```python
from build123d import *

# Parameters (mm, degrees)
F1_DEPTH = 4
F3_DEPTH = 2.5
F4_R     = 4
F5_DEPTH = 1
F6_R     = 1.75
F7_DEPTH = 5.001
F8_SIZE  = 0.99999


# Not quite as in the source:
# - a fillet or chamfer is up to 0.001 mm smaller than in the source, because OpenCascade refuses the exact size


with BuildPart() as f1:
    # F0 (on Top) → F1 (new body)
    with BuildSketch(Plane.XY):
        with BuildLine():
            ThreePointArc((-1.75, 7.5042031676), (-1.8060506469, 7.3388969595), (-1.9510840407, 7.2417726467))
            ThreePointArc((-1.9510840407, 7.2417726467), (-3.75, 6.4951905284), (-5.2960170601, 5.3105746675))
            ThreePointArc((-5.2960170601, 5.3105746675), (-5.4526458792, 5.2335342205), (-5.6238305783, 5.2676460404))
            Line((-5.6238305783, 5.2676460404), (-5.7871696323, 5.3619498872))
            ThreePointArc((-5.7871696323, 5.3619498872), (-6.3349564147, 5.8273689108), (-6.682813556, 6.4564004169))
            ThreePointArc((-6.682813556, 6.4564004169), (-12.124355653, 7), (-8.932813556, 2.5592860998))
            ThreePointArc((-8.932813556, 2.5592860998), (-8.2141277213, 2.5725487316), (-7.5371696323, 2.330860974))
            Line((-7.5371696323, 2.330860974), (-7.3738305783, 2.2365571272))
            ThreePointArc((-7.3738305783, 2.2365571272), (-7.2586965261, 2.105362739), (-7.2471011008, 1.9311979792))
            ThreePointArc((-7.2471011008, 1.9311979792), (-7.5, 0), (-7.2471011008, -1.9311979792))
            ThreePointArc((-7.2471011008, -1.9311979792), (-7.2586965261, -2.105362739), (-7.3738305783, -2.2365571272))
            Line((-7.3738305783, -2.2365571272), (-7.5371696323, -2.330860974))
            ThreePointArc((-7.5371696323, -2.330860974), (-8.2141277213, -2.5725487316), (-8.932813556, -2.5592860998))
            ThreePointArc((-8.932813556, -2.5592860998), (-12.124355653, -7), (-6.682813556, -6.4564004169))
            ThreePointArc((-6.682813556, -6.4564004169), (-6.3349564147, -5.8273689108), (-5.7871696323, -5.3619498872))
            Line((-5.7871696323, -5.3619498872), (-5.6238305783, -5.2676460404))
            ThreePointArc((-5.6238305783, -5.2676460404), (-5.4526458792, -5.2335342205), (-5.2960170601, -5.3105746675))
            ThreePointArc((-5.2960170601, -5.3105746675), (-3.75, -6.4951905284), (-1.9510840407, -7.2417726467))
            ThreePointArc((-1.9510840407, -7.2417726467), (-1.8060506469, -7.3388969595), (-1.75, -7.5042031676))
            Line((-1.75, -7.5042031676), (-1.75, -7.6928108612))
            ThreePointArc((-1.75, -7.6928108612), (-1.8791713066, -8.3999176424), (-2.25, -9.0156865167))
            ThreePointArc((-2.25, -9.0156865167), (0, -14), (2.25, -9.0156865167))
            ThreePointArc((2.25, -9.0156865167), (1.8791713066, -8.3999176424), (1.75, -7.6928108612))
            Line((1.75, -7.6928108612), (1.75, -7.5042031676))
            ThreePointArc((1.75, -7.5042031676), (1.8060506469, -7.3388969595), (1.9510840407, -7.2417726467))
            ThreePointArc((1.9510840407, -7.2417726467), (3.75, -6.4951905284), (5.2960170601, -5.3105746675))
            ThreePointArc((5.2960170601, -5.3105746675), (5.4526458792, -5.2335342205), (5.6238305783, -5.2676460404))
            Line((5.6238305783, -5.2676460404), (5.7871696323, -5.3619498872))
            ThreePointArc((5.7871696323, -5.3619498872), (6.3349564147, -5.8273689108), (6.682813556, -6.4564004169))
            ThreePointArc((6.682813556, -6.4564004169), (12.124355653, -7), (8.932813556, -2.5592860998))
            ThreePointArc((8.932813556, -2.5592860998), (8.2141277213, -2.5725487316), (7.5371696323, -2.330860974))
            Line((7.5371696323, -2.330860974), (7.3738305783, -2.2365571272))
            ThreePointArc((7.3738305783, -2.2365571272), (7.2586965261, -2.105362739), (7.2471011008, -1.9311979792))
            ThreePointArc((7.2471011008, -1.9311979792), (7.5, 0), (7.2471011008, 1.9311979792))
            ThreePointArc((7.2471011008, 1.9311979792), (7.2586965261, 2.105362739), (7.3738305783, 2.2365571272))
            Line((7.3738305783, 2.2365571272), (7.5371696323, 2.330860974))
            ThreePointArc((7.5371696323, 2.330860974), (8.2141277213, 2.5725487316), (8.932813556, 2.5592860998))
            ThreePointArc((8.932813556, 2.5592860998), (12.124355653, 7), (6.682813556, 6.4564004169))
            ThreePointArc((6.682813556, 6.4564004169), (6.3349564147, 5.8273689108), (5.7871696323, 5.3619498872))
            Line((5.7871696323, 5.3619498872), (5.6238305783, 5.2676460404))
            ThreePointArc((5.6238305783, 5.2676460404), (5.4526458792, 5.2335342205), (5.2960170601, 5.3105746675))
            ThreePointArc((5.2960170601, 5.3105746675), (3.75, 6.4951905284), (1.9510840407, 7.2417726467))
            ThreePointArc((1.9510840407, 7.2417726467), (1.8060506469, 7.3388969595), (1.75, 7.5042031676))
            Line((1.75, 7.5042031676), (1.75, 7.6928108612))
            ThreePointArc((1.75, 7.6928108612), (1.8791713066, 8.3999176424), (2.25, 9.0156865167))
            ThreePointArc((2.25, 9.0156865167), (0, 14), (-2.25, 9.0156865167))
            ThreePointArc((-2.25, 9.0156865167), (-1.8791713066, 8.3999176424), (-1.75, 7.6928108612))
            Line((-1.75, 7.6928108612), (-1.75, 7.5042031676))
        make_face()
    extrude(amount=F1_DEPTH)

    # F2 (on Top) → F3 (cut)
    with BuildSketch(Plane.XY):
        Polygon((2.875, -1.6598820239), (2.875, 1.6598820239), (0, 3.3197640478), (-2.875, 1.6598820239), (-2.875, -1.6598820239), (0, -3.3197640478), align=None)
    extrude(amount=F3_DEPTH, mode=Mode.SUBTRACT)

    # F4 (on face) → F5 (join)
    with BuildSketch(Plane.XY.offset(4)):
        Circle(F4_R)
    extrude(amount=F5_DEPTH)

    # F6 (on face) → F7 (cut, through all)
    with BuildSketch(Plane.XY.offset(5)):
        Circle(F6_R)
    extrude(amount=-F7_DEPTH, mode=Mode.SUBTRACT)

    # F8 (size 1 in the source; OpenCascade refuses exactly that, so slightly less here)
    f8_edges = [f1.edges().sort_by_distance(p)[0] for p in [
        (1.75, -7.598507, 4),
        (1.879171, -8.399918, 4),
        (1.806051, -7.338897, 4),
        (0, -14, 4),
        (3.75, -6.495191, 4),
        (-1.879171, -8.399918, 4),
        (5.452646, -5.233534, 4),
        (-1.75, -7.598507, 4),
        (5.7055, -5.314798, 4),
        (-1.806051, -7.338897, 4),
        (6.334956, -5.827369, 4),
        (-3.75, -6.495191, 4),
        (12.124356, -7, 4),
        (-5.452646, -5.233534, 4),
        (8.214128, -2.572549, 4),
        (-5.7055, -5.314798, 4),
        (7.4555, -2.283709, 4),
        (-6.334956, -5.827369, 4),
        (7.258697, -2.105363, 4),
        (-12.124356, -7, 4),
        (7.5, 0, 4),
        (-8.214128, -2.572549, 4),
        (7.258697, 2.105363, 4),
        (-7.4555, -2.283709, 4),
        (7.4555, 2.283709, 4),
        (-7.258697, -2.105363, 4),
        (8.214128, 2.572549, 4),
        (-7.5, 0, 4),
        (12.124356, 7, 4),
        (-7.258697, 2.105363, 4),
        (6.334956, 5.827369, 4),
        (-7.4555, 2.283709, 4),
        (5.7055, 5.314798, 4),
        (-8.214128, 2.572549, 4),
        (5.452646, 5.233534, 4),
        (-12.124356, 7, 4),
        (3.75, 6.495191, 4),
        (-6.334956, 5.827369, 4),
        (1.806051, 7.338897, 4),
        (-5.7055, 5.314798, 4),
        (1.75, 7.598507, 4),
        (-5.452646, 5.233534, 4),
        (1.879171, 8.399918, 4),
        (-3.75, 6.495191, 4),
        (0, 14, 4),
        (-1.806051, 7.338897, 4),
        (-1.879171, 8.399918, 4),
        (-1.75, 7.598507, 4),
        (-4, 0, 4),
        (-12.124356, -7, 0),
    ]]
    chamfer(f8_edges, length=F8_SIZE)


solid = f1.part
```
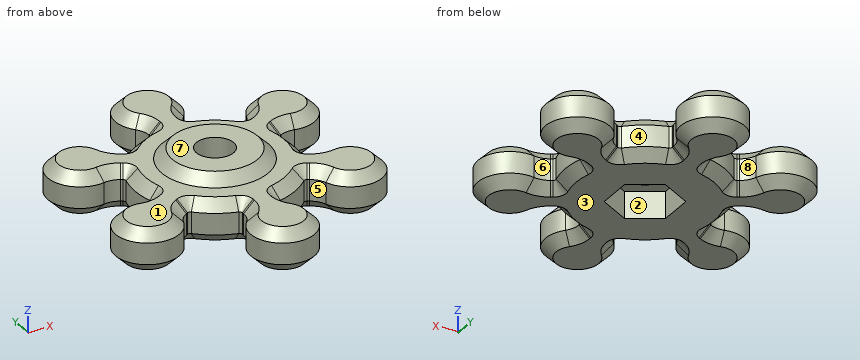
The model under review builds one solid part; all positions refer to its coordinate system, in mm. Face numbers are marked on the shaded views. A direction names the side the tool comes from. Coordinates: 2 decimals unless noted, no trailing zeros. Write each loop counter-clockwise with the first axis right and the second up, starting at its lowest first coordinate (ties: lowest second). Pieces come first, ordered by that corner, then holes.
1) The part is to be moulded in two halves that separate along Y. For the marked faces 6, 7 and 8, say which applies: pulls with the +Y half, pulls with the -Y half, needs draft (parallel to the pull), parting line crosses it, or undercut.
2) We need section B-B on y = -11. State the section outline as (x, z) points, then the cut area to 3 significant figures.
3) To check wall thickness, follow probe 1 along Y at (x, z) = (2.5, 1.8); probe 2 along Y at (x, z) = (0, 4.5); probe 3 along X at (y, z) = (-6.25, 0.7). State the ranges of each line that lie inside material, in increasing order.
4) Clearance check with flat-ended pins moving along their axes: pin 1 Ø3 at (y, z) = (0, 1) entering from +X; pin 2 Ø1.2 at (y, z) = (0.5, 2) entering from -X; pin 3 Ø4 at (x, y) = (-8, -7.5) entering from +Z. State where each tip first meets the part, or that it passes through.
5) Machinability: for the marked faces 1, 2, 3, 4 and 5, which of the approach directions +Z, -Z, +X, -X, +Y, -Y give a long, thin tool a straight path to every point of the face, cutting with its end or side? Answer none if there is none.
Answer list:
1. face 6: undercut
1. face 7: needs draft
1. face 8: pulls with the +Y half
2. outline: (-3, 1) - (-2, 0) - (2, 0) - (3, 1) - (3, 3) - (2, 4) - (-2, 4) - (-3, 3) - close
2. area: 22.0 mm2
3. probe 1: y = -12.66 to -9.34, -7.07 to -1.88, 1.88 to 7.07, 9.34 to 12.66
3. probe 2: y = -4.5 to -1.75, 1.75 to 4.5
3. probe 3: x = -12.12 to -6.93, -3.57 to 3.57, 6.93 to 12.12
4. pin 1: stops at x = 7.5
4. pin 2: stops at x = -7.5
4. pin 3: stops at z = 4
5. face 1: +Z
5. face 2: -Z
5. face 3: -Z, +X, -X, +Y, -Y
5. face 4: +Z, -Z
5. face 5: +Z, -Z, -Y
